Drawing for the job (mm, zero at the part's lowest x, y, z). A direction names the side the tool comes from. Give positions to 0.01 mm unless a question says otherwise; leave off trailing zeros. Order: outer loops, then holes, each group sorted by start corner. A loop starts at its lowest first (then second) coordinate and runs counter-clockwise, first axis right, second up. Notation, with made-up numbers: M 6.5,13.25 L 52.5,13.25 A22 cw 52.5,20.25 Z; hole C 67,-11 d10. An arc over 180 degrees is marked long. One line per item, written item: value.
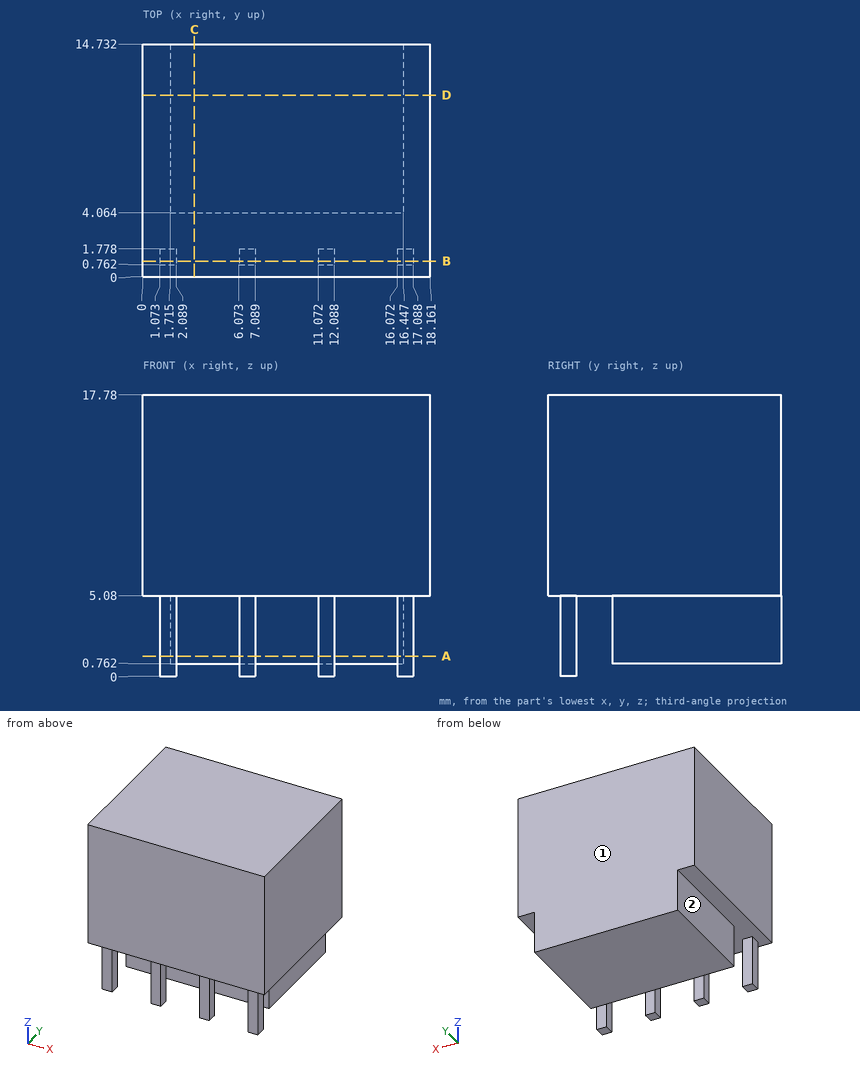
1) Saw through at C-C, the plane x = 3.25. Write the cut outline in (y, z) (1 decimal).
Check values:
outline: M 0,5.1 L 4.1,5.1 L 4.1,0.8 L 14.7,0.8 L 14.7,17.8 L 0,17.8 Z
2) Drill centre lines: probe 1 along Z at (x, y) = (13.75, 3); probe 2 along Z at (x, y) = (9.25, 6); probe 3 along X at (y, z) = (11.25, 3.5) (1 decimal). Where is each one in solid material? Low to high. Write a range as from..to.
Check values:
probe 1: 5.08..17.78
probe 2: 0.76..17.78
probe 3: 1.7..16.4
3) Pin check, flat tips, straight feed: pin 1 (3.5 mm diameter, centred on y = 7.5, z = 3, fed in from +X); pin 2 (0.5 mm diameter, centred on y = 1, z = 2, fed in from -X); pin 3 (1.1 mm diameter, centred on x = 16.5, z = 2, fed in from +Y); pin 4 (1.1 mm diameter, centred on y = 1.5, z = 2, fed in from +X). Stop position of each tip, or through.
Check values:
pin 1: x = 16.45
pin 2: x = 1.07
pin 3: y = 14.73
pin 4: x = 17.09
4) Saw through at A-A, the plane z = 1.25. Write the cut outline in (x, y) (1 decimal), then the cut area to 3 significant figures.
Check values:
outline: M 1.1,0.8 L 2.1,0.8 L 2.1,1.8 L 1.1,1.8 Z; M 1.7,4.1 L 16.4,4.1 L 16.4,14.7 L 1.7,14.7 Z; M 6.1,0.8 L 7.1,0.8 L 7.1,1.8 L 6.1,1.8 Z; M 11.1,0.8 L 12.1,0.8 L 12.1,1.8 L 11.1,1.8 Z; M 16.1,0.8 L 17.1,0.8 L 17.1,1.8 L 16.1,1.8 Z
area: 161 mm^2
5) Saw through at B-B, the plane y = 1. Write the cut outline in (x, z), then the cut area to 3 significant figures.
Check values:
outline: M 0,5.08 L 1.07,5.08 L 1.07,0 L 2.09,0 L 2.09,5.08 L 6.07,5.08 L 6.07,0 L 7.09,0 L 7.09,5.08 L 11.07,5.08 L 11.07,0 L 12.09,0 L 12.09,5.08 L 16.07,5.08 L 16.07,0 L 17.09,0 L 17.09,5.08 L 18.16,5.08 L 18.16,17.78 L 0,17.78 Z
area: 251 mm^2
6) Saw through at D-D, the plane y = 11.5. Write the cut outline in (x, z) (1 decimal), then the cut area to 3 significant figures.
Check values:
outline: M 0,5.1 L 1.7,5.1 L 1.7,0.8 L 16.4,0.8 L 16.4,5.1 L 18.2,5.1 L 18.2,17.8 L 0,17.8 Z
area: 294 mm^2
7) Tool access for the marked faces 1 and 2: list every direction of +Z, -Z, +X, -X, +Y, -Y with a clear straight run to the whole face (end or side of a thin tool).
Check values:
face 1: +Z, -Z, +X, -X, +Y
face 2: -Z, -X, +Y
